Read the model definition and answer for the solid it produces. Units are mm, in the model's axes. A direction names the side the tool comes from. Coordinates: 2 decimals unless noted, no trailing zeros. Write each loop counter-clockwise with the first axis right and the second up, starting at its lowest first coordinate (ties: lowest second). Pieces come first, ordered by that corner, then holes. Notation, with made-up numbers: (-14.75, 52) - (-7.75, 52) arc R14 ccw to (-7.75, 71) - close; hole circle Ø5 at (34.5, 66). An arc over 180 degrees is marked (long way). Return JSON: item names as keys, results as strings.
```python
from build123d import *

# Parameters (mm, degrees)
BOSS_EXTRUDE1_DEPTH = 10
BOSS_EXTRUDE2_DEPTH = 1
SKETCH4_R           = 5
CUT_EXTRUDE1_DEPTH  = 68.330244319


with BuildPart() as part:
    # Sketch2 → Boss-Extrude1 (new body)
    with BuildSketch(Plane(origin=(0, 0, 0), x_dir=(1, 0, 0), z_dir=(0, 1, 0))):
        with BuildLine():
            Line((-8.33, 46.225447537), (-8.33, 34.685513519))
            ThreePointArc((-8.33, 34.685513519), (0, -35.67175), (8.33, 34.685513519))
            Line((8.33, 34.685513519), (8.33, 46.225447537))
            ThreePointArc((8.33, 46.225447537), (0, -46.97), (-8.33, 46.225447537))
        make_face()
    extrude(amount=BOSS_EXTRUDE1_DEPTH)

    # Sketch3 → Boss-Extrude2 (add)
    with BuildSketch(Plane(origin=(0, 10, 0), x_dir=(1, 0, 0), z_dir=(0, 1, 0))):
        with BuildLine():
            Line((-8.33, 46.225447537), (-8.33, 22.985447537))
            Line((-8.33, 22.985447537), (8.33, 22.985447537))
            Line((8.33, 22.985447537), (8.33, 46.225447537))
            ThreePointArc((8.33, 46.225447537), (0, -46.97), (-8.33, 46.225447537))
        make_face()
    extrude(amount=BOSS_EXTRUDE2_DEPTH)

    # Sketch4 → Cut-Extrude1 (cut, through all)
    with BuildSketch(Plane(origin=(0, 11, 0), x_dir=(1, 0, 0), z_dir=(0, 1, 0))):
        with Locations(Location((8.605489527, -8.605489527, 0), (0, 0, 270))):
            Circle(SKETCH4_R)
    extrude(amount=-CUT_EXTRUDE1_DEPTH, mode=Mode.SUBTRACT)


solid = part.part
```
(1) Straight lines are drawn through the part: line 1 (X direction, y = 4.75, z = 0); line 2 (Y direction, x = 12, z = -14); line 3 (X direction, y = 8, z = -29.5). For each, find the intervals that lie inside material, in ascending order. Write a range as from..to.
Answer:
{"line 1": "-46.97..-35.67, 35.67..46.97", "line 2": "10..11", "line 3": "-36.55..-20.06, 20.06..36.55"}
(2) A cutting plane is placed at A-A (z = -39.5). Determine the outline of the cut face in (x, y).
Answer:
{"outline": "(-25.42, 0) - (-8.33, 0) - (-8.33, 11) - (-25.42, 11) - close; (8.33, 0) - (25.42, 0) - (25.42, 11) - (8.33, 11) - close"}
(3) A cutting plane is placed at B-B (x = 0). Determine the outline of the cut face in (y, z), and give its area (3 significant figures).
Answer:
{"outline": "(0, 35.67) - (10, 35.67) - (10, -22.99) - (11, -22.99) - (11, 46.97) - (0, 46.97) - close", "area": "183 mm²"}
(4) A cutting plane is placed at C-C (z = 0). Determine the outline of the cut face in (x, y), and give its area (3 significant figures).
Answer:
{"outline": "(-46.97, 0) - (-35.67, 0) - (-35.67, 10) - (35.67, 10) - (35.67, 0) - (46.97, 0) - (46.97, 11) - (-46.97, 11) - close", "area": "320 mm²"}
(5) Determine the mould class of faces 1 (the face through (13.563, 10.507, 7.955)), 2 (the face through (1.95, 5.42, 46.93)), 3 (the face through (1, 11, 0)) for opening direction X: +X half, -X half, draft (parallel to the pull), parting line (faces both ways), or undercut.
Answer:
{"face 1": "undercut", "face 2": "parting line", "face 3": "draft"}
(6) A cutting plane is placed at D-D (y = 3). Determine the outline of the cut face in (x, z), and give its area (3 significant figures).
Answer:
{"outline": "(-8.33, -46.23) - (-8.33, -34.69) arc R35.67 cw (long way) to (8.33, -34.69) - (8.33, -46.23) arc R46.97 ccw (long way) to start", "area": "2,740 mm²"}
(7) Which of the six approach directions +Z, -Z, +X, -X, +Y, -Y give full straight-line access (tool end or side, diameter ignored) to faces 4 (the face through (18, 0, 31)), 5 (the face through (8.33, 5, -40)), 6 (the face through (0, 10, 0))?
Answer:
{"face 4": "+Z, -Z, +X, -X, -Y", "face 5": "-Z, +Y, -Y", "face 6": "-Y"}
(8) Flat-ended cylindrical pins translate along their axes: P1, Ø5, axis at y = 9, z = 8, coming from the -X side; P2, Ø6, axis at x = 23, y = 2.5, coming from the +Z side; P3, Ø2, axis at x = 5.5, y = 1.5, coming from the +Z side; P4, Ø8, axis at x = 8.61, z = 8.61, coming from the +Y side. Find the tip coordinate at first contact, or state that the pin passes through.
Answer:
{"P1": "x = -46.65", "P2": "z = 42.5", "P3": "z = 46.75", "P4": "through"}
